```python
from build123d import *

# Parameters (mm, degrees)
SKETCH1_W           = 450
SKETCH1_H           = 300
BOSS_EXTRUDE1_DEPTH = 70
CUT_EXTRUDE1_DEPTH  = 451
SKETCH3_R           = 25
BOSS_EXTRUDE2_DEPTH = 58
BOSS_EXTRUDE3_DEPTH = 20
SKETCH5_R           = 25
REVOLVE1_ANGLE      = 180


with BuildPart() as part:
    # Sketch1 → Boss-Extrude1 (new body)
    with BuildSketch(Plane(origin=(0, 0, 0), x_dir=(1, 0, 0), z_dir=(0, 1, 0))):
        Rectangle(SKETCH1_W, SKETCH1_H)
    extrude(amount=BOSS_EXTRUDE1_DEPTH)

    # Sketch2 → Cut-Extrude1 (cut, through all)
    with BuildSketch(Plane(origin=(225, 0, 0), x_dir=(0, 0, -1), z_dir=(1, 0, 0))):
        Polygon((-60, 0), (-42.679491924, 30), (42.679491924, 30), (60, 0), align=None)
    extrude(amount=-CUT_EXTRUDE1_DEPTH, mode=Mode.SUBTRACT)

    # Sketch3 → Boss-Extrude2 (add)
    with BuildSketch(Plane(origin=(0, 70, 0), x_dir=(1, 0, 0), z_dir=(0, 1, 0))):
        with BuildLine():
            Line((-80, -88.110802776), (-80, 88.110802776))
            ThreePointArc((-80, 88.110802776), (-99.471105521, 99.337628307), (-117.391304348, 112.903469074))
            ThreePointArc((-117.391304348, 112.903469074), (-186.051805285, 109.644874595), (-186.576083953, 40.909090909))
            ThreePointArc((-186.576083953, 40.909090909), (-170.467384697, 0), (-186.576083953, -40.909090909))
            ThreePointArc((-186.576083953, -40.909090909), (-186.051805285, -109.644874595), (-117.391304348, -112.903469074))
            ThreePointArc((-117.391304348, -112.903469074), (-99.471105521, -99.337628307), (-80, -88.110802776))
        make_face()
        with Locations((-150, -75)):
            Circle(SKETCH3_R, mode=Mode.SUBTRACT)
        with Locations((-150, 75)):
            Circle(SKETCH3_R, mode=Mode.SUBTRACT)
        with BuildLine():
            ThreePointArc((80, 88.110802776), (0, 69.355957742), (-80, 88.110802776))
            Line((-80, 88.110802776), (-80, -88.110802776))
            ThreePointArc((-80, -88.110802776), (0, -69.355957742), (80, -88.110802776))
            Line((80, -88.110802776), (80, 88.110802776))
        make_face()
        with BuildLine():
            ThreePointArc((117.391304348, 112.903469074), (99.471105521, 99.337628307), (80, 88.110802776))
            Line((80, 88.110802776), (80, -88.110802776))
            ThreePointArc((80, -88.110802776), (99.471105521, -99.337628307), (117.391304348, -112.903469074))
            ThreePointArc((117.391304348, -112.903469074), (186.051805285, -109.644874595), (186.576083953, -40.909090909))
            ThreePointArc((186.576083953, -40.909090909), (170.467384697, 0), (186.576083953, 40.909090909))
            ThreePointArc((186.576083953, 40.909090909), (186.051805285, 109.644874595), (117.391304348, 112.903469074))
        make_face()
        with Locations((150, -75)):
            Circle(SKETCH3_R, mode=Mode.SUBTRACT)
        with Locations((150, 75)):
            Circle(SKETCH3_R, mode=Mode.SUBTRACT)
        with Locations((-150, 75)):
            Circle(SKETCH3_R)
        with Locations((-150, -75)):
            Circle(SKETCH3_R)
        with Locations((150, -75)):
            Circle(SKETCH3_R)
        with Locations((150, 75)):
            Circle(SKETCH3_R)
    extrude(amount=BOSS_EXTRUDE2_DEPTH)

    # Sketch4 → Boss-Extrude3 (add)
    with BuildSketch(Plane(origin=(0, 128, 0), x_dir=(1, 0, 0), z_dir=(0, 1, 0))):
        with BuildLine():
            Line((-80, 88.110802776), (-80, -88.110802776))
            ThreePointArc((-80, -88.110802776), (0, -69.355957742), (80, -88.110802776))
            Line((80, -88.110802776), (80, 88.110802776))
            ThreePointArc((80, 88.110802776), (0, 69.355957742), (-80, 88.110802776))
        make_face()
    extrude(amount=BOSS_EXTRUDE3_DEPTH)

    # Sketch5 → Revolve1 (revolve)
    with BuildSketch(Plane(origin=(0, 128, 0), x_dir=(1, 0, 0), z_dir=(0, 1, 0))):
        with Locations((-150, 75)):
            Circle(SKETCH5_R)
        with Locations((150, 75)):
            Circle(SKETCH5_R)
    revolve(axis=Axis((-226.209198956, 128, 0), (1, 0, 0)), revolution_arc=REVOLVE1_ANGLE)


solid = part.part
```
The model under review builds one solid part; all positions refer to its coordinate system, in mm. A direction names the side the tool comes from. Give positions to 0.01 mm unless a question says otherwise; leave off trailing zeros. Write each loop counter-clockwise with the first axis right and the second up, starting at its lowest first coordinate (ties: lowest second). Pieces come first, ordered by that corner, then holes. Notation, with made-up numbers: M -6,-19 L 44,-19 A25 ccw 44,4 Z; hole C -24,56 d7. An arc over 180 degrees is marked long. Answer in a Markdown table with one row per item.
Item 1: For P1, Ø3, axis at x = -45, z = -23, coming from the +Y side; P2, Ø10, axis at y = 141.5, z = 27, coming from the -X side; P3, Ø8, axis at x = 47.5, z = -28, coming from the -Y side, all flat-tipped, find the tip position at first contact; note any pin that passes through.
Check sheet entries:
| item | result |
|---|---|
| P1 | y = 148 |
| P2 | x = -80 |
| P3 | y = 30 |
Item 2: Add section C-C on y = 17.5. Give the boundary of the cut face in (x, z).
Check sheet entries:
| item | result |
|---|---|
| outline | M -225,-150 L 225,-150 L 225,-49.9 L -225,-49.9 Z; M -225,49.9 L 225,49.9 L 225,150 L -225,150 Z |
Item 3: Add section A-A on x = 150. Give the boundary of the cut face in (y, z), plus the area to 3 significant figures.
Check sheet entries:
| item | result |
|---|---|
| outline | M 0,-150 L 70,-150 L 70,-125 L 128,-125 L 128,-100 A100 ccw 128,100 L 128,125 L 70,125 L 70,150 L 0,150 L 0,60 L 30,42.68 L 30,-42.68 L 0,-60 Z; hole M 128,-50 A50 ccw 128,50 Z |
| area | 44,200 mm2 |
Item 4: Add section D-D on x = -70. Give the boundary of the cut face in (y, z), plus the area to 3 significant figures.
Check sheet entries:
| item | result |
|---|---|
| outline | M 0,-150 L 70,-150 L 70,-83.52 L 148,-83.52 L 148,83.52 L 70,83.52 L 70,150 L 0,150 L 0,60 L 30,42.68 L 30,-42.68 L 0,-60 Z |
| area | 30,900 mm2 |
Item 5: Add section B-B on y = 77. Give the boundary of the cut face in (x, z), plus the area to 3 significant figures.
Check sheet entries:
| item | result |
|---|---|
| outline | M -186.58,-40.91 A50 ccw -117.39,-112.9 A180 cw 117.39,-112.9 A50 ccw 186.58,-40.91 A60 cw 186.58,40.91 A50 ccw 117.39,112.9 A180 cw -117.39,112.9 A50 ccw -186.58,40.91 A60 cw Z |
| area | 73,100 mm2 |
Item 6: Tool access review of faces 1 (the face through (3.15, 14.79, 51.46)), 2 (the face through (-186.78, 98.59, 108.87)), 3 (the face through (1.79, 108.454, -69.365)): name each direction out of +Z, -Z, +X, -X, +Y, -Y from which nothing blocks a thin tool from reaching the whole face with its end or side.
Check sheet entries:
| item | result |
|---|---|
| face 1 | +X, -X, -Y |
| face 2 | +Y |
| face 3 | -Z, +Y |
Item 7: Draft analysis for pull direction X (two halves, no side actions). For faces 4 (the face through (-80, 138, -1)), 5 (the face through (3, 30, 1)), 6 (the face through (225, 35, 2)), state which applies: +X half, -X half, draft (parallel to the pull), parting line (faces both ways), or undercut.
Check sheet entries:
| item | result |
|---|---|
| face 4 | undercut |
| face 5 | draft |
| face 6 | +X half |
Item 8: For line 1 along Y through (x, z) = (-59, -63); line 2 along Y through (x, z) = (-11.5, -71); line 3 along Z through (x, y) = (3, 144), list the stretches that pass through material, from the lowest coordinate up.
Check sheet entries:
| item | result |
|---|---|
| line 1 | 0 to 148 |
| line 2 | 0 to 70 |
| line 3 | -69.38 to 69.38 |
